Verification items for the finished model (mm, model axes). Give positions to 0.01 mm unless a question says otherwise; leave off trailing zeros. Order: outer loops, then holes, each group sorted by start corner. A loop starts at its lowest first (then second) coordinate and runs counter-clockwise, first axis right, second up. Notation, with made-up numbers: (24.25, 45.5) -> (45.25, 45.5) arc R20 cw to (45.25, 65.5) -> close; hole circle Ø4 at (-30.5, -12). An arc over 180 degrees is marked (long way). Return JSON: item names as keys, results as strings. Group by question number.
(1) Cross-section at A-A on x = 0. Enter the section's corners in (y, z), then the cut area to 3 significant figures.
(2) Thickness scan on line 1 along X through (y, z) = (15, 102); line 2 along Y through (x, z) = (-19, 238.5); line 3 along Y through (x, z) = (0, 304). Record the ranges inside material, lowest first.
(3) Depth check by flat-ended pin: pin 1 Ø1 at (x, z) = (-2, 153.5) entering from -Y; pin 2 Ø5 at (x, y) = (13, -14) entering from +Z. Enter the tip coordinate at first touch or a pass-through.
(4) Cross-section at C-C on z = 35. State how many separate pieces and enclosed holes the cut face has, then the cut area to 3 significant figures.
from build123d import *

# Parameters (mm, degrees)
SKETCH1_R           = 5
BOSS_EXTRUDE1_DEPTH = 390


with BuildPart() as part:
    # Sketch1 → Boss-Extrude1 (new body)
    with BuildSketch(Plane.XY):
        with BuildLine():
            Line((-5, -15.705854984), (-8, -15.705854984))
            Line((-8, -15.705854984), (-8, -11.948495671))
            ThreePointArc((-8, -11.948495671), (-7.771638598, -10.800445374), (-7.121320344, -9.827175327))
            Line((-7.121320344, -9.827175327), (-4.66838954, -7.374244523))
            ThreePointArc((-4.66838954, -7.374244523), (-4.125357909, -7.094903463), (-3.52114023, -7.183423382))
            ThreePointArc((-3.52114023, -7.183423382), (0, -8), (3.52114023, -7.183423382))
            ThreePointArc((3.52114023, -7.183423382), (4.125357909, -7.094903463), (4.66838954, -7.374244523))
            Line((4.66838954, -7.374244523), (7.121320344, -9.827175327))
            ThreePointArc((7.121320344, -9.827175327), (7.771638598, -10.800445374), (8, -11.948495671))
            Line((8, -11.948495671), (8, -15.705854984))
            Line((8, -15.705854984), (5, -15.705854984))
            Line((5, -15.705854984), (5, -21.5))
            ThreePointArc((5, -21.5), (5.292893219, -22.207106781), (6, -22.5))
            Line((6, -22.5), (20.5, -22.5))
            ThreePointArc((20.5, -22.5), (21.914213562, -21.914213562), (22.5, -20.5))
            Line((22.5, -20.5), (22.5, -6))
            ThreePointArc((22.5, -6), (22.207106781, -5.292893219), (21.5, -5))
            Line((21.5, -5), (15.705854984, -5))
            Line((15.705854984, -5), (15.705854984, -8))
            Line((15.705854984, -8), (11.948495671, -8))
            ThreePointArc((11.948495671, -8), (10.800445374, -7.771638598), (9.827175327, -7.121320344))
            Line((9.827175327, -7.121320344), (7.374244523, -4.66838954))
            ThreePointArc((7.374244523, -4.66838954), (7.094903463, -4.125357909), (7.183423382, -3.52114023))
            ThreePointArc((7.183423382, -3.52114023), (8, 0), (7.183423382, 3.52114023))
            ThreePointArc((7.183423382, 3.52114023), (7.094903463, 4.125357909), (7.374244523, 4.66838954))
            Line((7.374244523, 4.66838954), (9.827175327, 7.121320344))
            ThreePointArc((9.827175327, 7.121320344), (10.800445374, 7.771638598), (11.948495671, 8))
            Line((11.948495671, 8), (15.705854984, 8))
            Line((15.705854984, 8), (15.705854984, 5))
            Line((15.705854984, 5), (21.5, 5))
            ThreePointArc((21.5, 5), (22.207106781, 5.292893219), (22.5, 6))
            Line((22.5, 6), (22.5, 20.5))
            ThreePointArc((22.5, 20.5), (21.914213562, 21.914213562), (20.5, 22.5))
            Line((20.5, 22.5), (6, 22.5))
            ThreePointArc((6, 22.5), (5.292893219, 22.207106781), (5, 21.5))
            Line((5, 21.5), (5, 15.705854984))
            Line((5, 15.705854984), (8, 15.705854984))
            Line((8, 15.705854984), (8, 11.948495671))
            ThreePointArc((8, 11.948495671), (7.771638598, 10.800445374), (7.121320344, 9.827175327))
            Line((7.121320344, 9.827175327), (4.66838954, 7.374244523))
            ThreePointArc((4.66838954, 7.374244523), (4.125357909, 7.094903463), (3.52114023, 7.183423382))
            ThreePointArc((3.52114023, 7.183423382), (0, 8), (-3.52114023, 7.183423382))
            ThreePointArc((-3.52114023, 7.183423382), (-4.125357909, 7.094903463), (-4.66838954, 7.374244523))
            Line((-4.66838954, 7.374244523), (-7.121320344, 9.827175327))
            ThreePointArc((-7.121320344, 9.827175327), (-7.771638598, 10.800445374), (-8, 11.948495671))
            Line((-8, 11.948495671), (-8, 15.705854984))
            Line((-8, 15.705854984), (-5, 15.705854984))
            Line((-5, 15.705854984), (-5, 21.5))
            ThreePointArc((-5, 21.5), (-5.292893219, 22.207106781), (-6, 22.5))
            Line((-6, 22.5), (-20.5, 22.5))
            ThreePointArc((-20.5, 22.5), (-21.914213562, 21.914213562), (-22.5, 20.5))
            Line((-22.5, 20.5), (-22.5, 6))
            ThreePointArc((-22.5, 6), (-22.207106781, 5.292893219), (-21.5, 5))
            Line((-21.5, 5), (-15.705854984, 5))
            Line((-15.705854984, 5), (-15.705854984, 8))
            Line((-15.705854984, 8), (-11.948495671, 8))
            ThreePointArc((-11.948495671, 8), (-10.800445374, 7.771638598), (-9.827175327, 7.121320344))
            Line((-9.827175327, 7.121320344), (-7.374244523, 4.66838954))
            ThreePointArc((-7.374244523, 4.66838954), (-7.094903463, 4.125357909), (-7.183423382, 3.52114023))
            ThreePointArc((-7.183423382, 3.52114023), (-8, 0), (-7.183423382, -3.52114023))
            ThreePointArc((-7.183423382, -3.52114023), (-7.094903463, -4.125357909), (-7.374244523, -4.66838954))
            Line((-7.374244523, -4.66838954), (-9.827175327, -7.121320344))
            ThreePointArc((-9.827175327, -7.121320344), (-10.800445374, -7.771638598), (-11.948495671, -8))
            Line((-11.948495671, -8), (-15.705854984, -8))
            Line((-15.705854984, -8), (-15.705854984, -5))
            Line((-15.705854984, -5), (-21.5, -5))
            ThreePointArc((-21.5, -5), (-22.207106781, -5.292893219), (-22.5, -6))
            Line((-22.5, -6), (-22.5, -20.5))
            ThreePointArc((-22.5, -20.5), (-21.914213562, -21.914213562), (-20.5, -22.5))
            Line((-20.5, -22.5), (-6, -22.5))
            ThreePointArc((-6, -22.5), (-5.292893219, -22.207106781), (-5, -21.5))
            Line((-5, -21.5), (-5, -15.705854984))
        make_face()
        Circle(SKETCH1_R, mode=Mode.SUBTRACT)
        with BuildLine():
            Line((-19, -21), (-7.5, -21))
            ThreePointArc((-7.5, -21), (-6.792893219, -20.707106781), (-6.5, -20))
            Line((-6.5, -20), (-6.5, -18.205854984))
            ThreePointArc((-6.5, -18.205854984), (-6.792893219, -17.498748202), (-7.5, -17.205854984))
            Line((-7.5, -17.205854984), (-8.5, -17.205854984))
            ThreePointArc((-8.5, -17.205854984), (-9.207106781, -16.912961765), (-9.5, -16.205854984))
            Line((-9.5, -16.205854984), (-9.5, -11.5))
            ThreePointArc((-9.5, -11.5), (-10.085786438, -10.085786438), (-11.5, -9.5))
            Line((-11.5, -9.5), (-16.205854984, -9.5))
            ThreePointArc((-16.205854984, -9.5), (-16.912961765, -9.207106781), (-17.205854984, -8.5))
            Line((-17.205854984, -8.5), (-17.205854984, -7.5))
            ThreePointArc((-17.205854984, -7.5), (-17.498748202, -6.792893219), (-18.205854984, -6.5))
            Line((-18.205854984, -6.5), (-20, -6.5))
            ThreePointArc((-20, -6.5), (-20.707106781, -6.792893219), (-21, -7.5))
            Line((-21, -7.5), (-21, -19))
            ThreePointArc((-21, -19), (-20.414213562, -20.414213562), (-19, -21))
        make_face(mode=Mode.SUBTRACT)
        with BuildLine():
            Line((-9.5, 16.205854984), (-9.5, 11.5))
            ThreePointArc((-9.5, 11.5), (-10.085786438, 10.085786438), (-11.5, 9.5))
            Line((-11.5, 9.5), (-16.205854984, 9.5))
            ThreePointArc((-16.205854984, 9.5), (-16.912961765, 9.207106781), (-17.205854984, 8.5))
            Line((-17.205854984, 8.5), (-17.205854984, 7.5))
            ThreePointArc((-17.205854984, 7.5), (-17.498748202, 6.792893219), (-18.205854984, 6.5))
            Line((-18.205854984, 6.5), (-20, 6.5))
            ThreePointArc((-20, 6.5), (-20.707106781, 6.792893219), (-21, 7.5))
            Line((-21, 7.5), (-21, 19))
            ThreePointArc((-21, 19), (-20.414213562, 20.414213562), (-19, 21))
            Line((-19, 21), (-7.5, 21))
            ThreePointArc((-7.5, 21), (-6.792893219, 20.707106781), (-6.5, 20))
            Line((-6.5, 20), (-6.5, 18.205854984))
            ThreePointArc((-6.5, 18.205854984), (-6.792893219, 17.498748202), (-7.5, 17.205854984))
            Line((-7.5, 17.205854984), (-8.5, 17.205854984))
            ThreePointArc((-8.5, 17.205854984), (-9.207106781, 16.912961765), (-9.5, 16.205854984))
        make_face(mode=Mode.SUBTRACT)
        with BuildLine():
            Line((16.205854984, 9.5), (11.5, 9.5))
            ThreePointArc((11.5, 9.5), (10.085786438, 10.085786438), (9.5, 11.5))
            Line((9.5, 11.5), (9.5, 16.205854984))
            ThreePointArc((9.5, 16.205854984), (9.207106781, 16.912961765), (8.5, 17.205854984))
            Line((8.5, 17.205854984), (7.5, 17.205854984))
            ThreePointArc((7.5, 17.205854984), (6.792893219, 17.498748202), (6.5, 18.205854984))
            Line((6.5, 18.205854984), (6.5, 20))
            ThreePointArc((6.5, 20), (6.792893219, 20.707106781), (7.5, 21))
            Line((7.5, 21), (19, 21))
            ThreePointArc((19, 21), (20.414213562, 20.414213562), (21, 19))
            Line((21, 19), (21, 7.5))
            ThreePointArc((21, 7.5), (20.707106781, 6.792893219), (20, 6.5))
            Line((20, 6.5), (18.205854984, 6.5))
            ThreePointArc((18.205854984, 6.5), (17.498748202, 6.792893219), (17.205854984, 7.5))
            Line((17.205854984, 7.5), (17.205854984, 8.5))
            ThreePointArc((17.205854984, 8.5), (16.912961765, 9.207106781), (16.205854984, 9.5))
        make_face(mode=Mode.SUBTRACT)
        with BuildLine():
            Line((9.5, -16.205854984), (9.5, -11.5))
            ThreePointArc((9.5, -11.5), (10.085786438, -10.085786438), (11.5, -9.5))
            Line((11.5, -9.5), (16.205854984, -9.5))
            ThreePointArc((16.205854984, -9.5), (16.912961765, -9.207106781), (17.205854984, -8.5))
            Line((17.205854984, -8.5), (17.205854984, -7.5))
            ThreePointArc((17.205854984, -7.5), (17.498748202, -6.792893219), (18.205854984, -6.5))
            Line((18.205854984, -6.5), (20, -6.5))
            ThreePointArc((20, -6.5), (20.707106781, -6.792893219), (21, -7.5))
            Line((21, -7.5), (21, -19))
            ThreePointArc((21, -19), (20.414213562, -20.414213562), (19, -21))
            Line((19, -21), (7.5, -21))
            ThreePointArc((7.5, -21), (6.792893219, -20.707106781), (6.5, -20))
            Line((6.5, -20), (6.5, -18.205854984))
            ThreePointArc((6.5, -18.205854984), (6.792893219, -17.498748202), (7.5, -17.205854984))
            Line((7.5, -17.205854984), (8.5, -17.205854984))
            ThreePointArc((8.5, -17.205854984), (9.207106781, -16.912961765), (9.5, -16.205854984))
        make_face(mode=Mode.SUBTRACT)
    extrude(amount=BOSS_EXTRUDE1_DEPTH)


solid = part.part
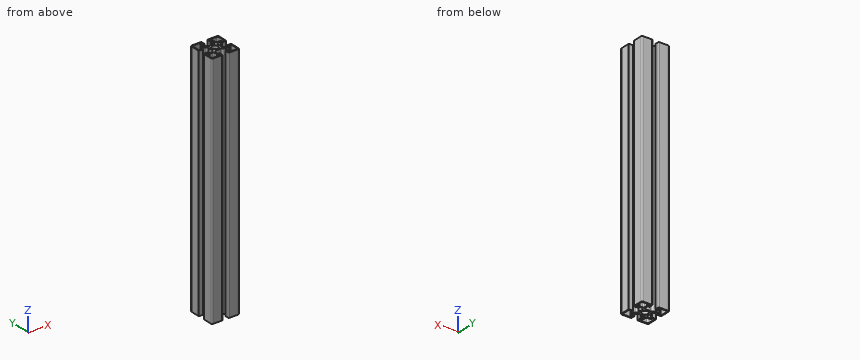
Verdict:
{
 "1": {"outline": "(-8, 0) -> (-5, 0) -> (-5, 390) -> (-8, 390) -> close; (5, 0) -> (8, 0) -> (8, 390) -> (5, 390) -> close", "area": "2,340 mm²"},
 "2": {"line 1": "-22.5 to -21, -9.5 to -8, 8 to 9.5, 21 to 22.5", "line 2": "-22.5 to -21, -6.5 to -5, 5 to 6.5, 21 to 22.5", "line 3": "-8 to -5, 5 to 8"},
 "3": {"pin 1": "y = -7.86", "pin 2": "through"},
 "4": {"separate pieces": "1", "enclosed holes": "5", "area": "579 mm²"}
}
